Autodesk Inventor part; units mm, degrees
ref_plane "Work Plane3" through (137.521, 56.9702, 137.521) normal (0.7071068, 0, 0.7071068) x (0, -1, 0)
ref_plane "YZ Plane" through (0, 0, 0) normal (1, 0, 0) x (0, 1, 0)
ref_plane "XZ Plane" through (0, 0, 0) normal (0, 1, 0) x (-1, 0, 0)
sketch "Sketch1" plane through (0, 0, 0) normal (0, 0, 1) x (1, 0, 0)
  line L0 (0, 0) -> (0, 228.6)
  line L1 (0, 228.6) -> (76.2, 228.6)
  line L2 (76.2, 228.6) -> (76.2, 219.2528)
  line L3 (76.2, 219.2528) -> (101.6, 219.2528)
  line L4 (101.6, 219.2528) -> (101.6, 0)
  line L5 (101.6, 0) -> (0, 0)
  dimension "d0" = 228.6
  dimension "d1" = 76.2
  dimension "d2" = 9.3472
  dimension "d3" = 25.4
extrude "Extrusion1" add sketch "Sketch1" along normal blind 812.8
sketch "Sketch6" plane through (0, 0, 0) normal (0, -1, 0) x (1, 0, 0)
  line L0 (101.6, 0) -> (101.6, 812.8)
  line L1 (0, 812.8) -> (101.6, 711.2)
  line L2 (76.2038, 736.5962) -> (25.4038, 736.5962)
  line L3 (25.4038, 736.5962) -> (25.4038, 787.3962)
  line L4 (25.4038, 787.3962) -> (76.2, 736.6)
  point P0 (0, 0)
  point P1 (101.6, 101.6)
  dimension "d31" = 35.9156
  dimension "d32" = 50.8
  dimension "d33" = 50.8
extrude "Extrusion4" cut sketch "Sketch6" against normal blind 181.1528
sketch "Sketch7" plane through (25.4038, 0, 736.5962) normal (0, -1, 0) x (1, 0, 0)
  line L0 (76.1962, -634.9962) -> (50.7962, -660.3962)
  line L1 (50.7962, -660.3962) -> (-0.0038, -660.3962)
  line L2 (76.1962, -634.9962) -> (-25.4038, -736.5962)
  line L3 (76.1962, -736.5962) -> (76.1962, 76.2038)
  line L4 (-0.0038, -660.3962) -> (-0.0038, -711.1962)
  line L5 (-0.0038, -711.1962) -> (50.7962, -660.3962)
  point P0 (76.1962, -25.3962)
  dimension "d39" = 50.8
  dimension "d41" = 90
  dimension "d42" = 50.8
extrude "Extrusion5" cut sketch "Sketch7" against normal blind 181.1528
chamfer "Chamfer5" distance 101.6 angle 45 1 edges at (101.6, 109.6264, 812.8)
chamfer "Chamfer6" distance 101.6 angle 45 1 edges at (101.6, 109.6264, 0)
ref_plane "Work Plane3" through (137.521, 56.9702, 137.521) normal (0.7071068, 0, 0.7071068) x (0, -1, 0)
sketch "Sketch9" plane through (137.521, 56.9702, 137.521) normal (0.7071068, 0, 0.7071068) x (0, -1, 0)
  line L0 (-162.2826, 0) -> (-162.2826, -466.9733)
  line L1 (-162.2826, 0) -> (-48.0842, 0)
  line L2 (-162.2826, 0) -> (56.9702, 0)
  dimension "d65" = 114.1984
hole "Hole2" at (137.521, 105.0544, 137.521) direction (-0.7071068, 0, -0.7071068) diameter 12.7 depth 127 tip angle 118
sketch "Sketch10" plane through (0, 181.1528, 0) normal (0, -1, 0) x (1, 0, 0)
  line L0 (76.2, 76.2) -> (76.2, 736.6)
  line L1 (76.2, 76.2) -> (63.5019, 63.5019)
  line L2 (0, 0) -> (76.2, 76.2)
  line L3 (63.5019, 63.5019) -> (38.1019, 63.5019)
  line L4 (38.1019, 63.5019) -> (38.1019, 38.1019)
  line L5 (63.5019, 63.5019) -> (38.1019, 38.1019)
  line L6 (76.2038, 736.5962) -> (63.5058, 749.2942)
  line L7 (63.5058, 749.2942) -> (38.1058, 749.2942)
  line L8 (38.1058, 749.2942) -> (38.1058, 774.6942)
  line L9 (63.5058, 749.2942) -> (38.1058, 774.6942)
  dimension "d73" = 17.9578
  dimension "d74" = 25.4
  dimension "d75" = 17.9578
  dimension "d76" = 25.4
extrude "Extrusion6" cut sketch "Sketch10" against normal blind 3.175 contours L7 L8 L9
sketch "Sketch11" plane through (25.4038, 181.1528, 736.5962) normal (0, -1, 0) x (1, 0, 0)
  line L0 (50.7962, -660.3962) -> (38.0981, -673.0942)
  line L1 (38.0981, -673.0942) -> (12.6962, -673.0942)
  line L2 (12.6962, -673.0942) -> (12.6962, -698.4962)
  line L3 (38.0981, -673.0942) -> (12.6962, -698.4962)
  line L4 (-25.4038, -736.5962) -> (50.7962, -660.3962)
  dimension "d79" = 17.9578
  dimension "d80" = 180
  dimension "d81" = 25.4019
  dimension "d82" = 25.4019
extrude "Extrusion7" cut sketch "Sketch11" against normal blind 3.175
properties part number "SideWidthOutlet" material "Wood (Birch)"
Work out the finished part from the listing and answer in its coordinate system (mm). A direction names the side the tool comes from. Give positions to 0.01 mm unless a question says otherwise; leave off trailing zeros. Loops run counter-clockwise (first coordinate to the right, second up) from the corner with the lowest first, then second, coordinate; pieces in that order, holes last. Notation, with made-up numbers: (73.25, 58) -> (95.25, 58) arc R15 ccw to (95.25, 69) -> close; hole circle Ø4 at (-40, 77.5). An arc over 180 degrees is marked (long way). Use a Markdown table: item, result. Add a question column.
1. Section B-B on x = 8.5 is taken. Determine the outline of the cut face in (y, z).
2. Find the intervals of material crossed by probe 1 along Z at (x, y) = (42.5, 117.5); probe 2 along Y at (x, z) = (92.5, 279.5); probe 3 along Z at (x, y) = (94.5, 90), in increasing order.
3. Flat-ended cylindrical pins translate along their axes: pin 1 Ø4 at (x, y) = (56, 122) entering from +Z; pin 2 Ø1.6 at (x, y) = (49, 182.5) entering from +Z; pin 3 Ø12.5 at (x, z) = (52.5, 45.5) entering from -Y. Find the tip coordinate at first contact, or state that the pin passes through.
4. Determine the mould class of faces 6 (the flat face through (25.4, 89, 51)), 7 (the cylindrical face through (84.17, 104.91, 93.15)), 8 (the flat face through (38, 228.6, 401)), 9 (the flat face through (52, 0, 401)) for opening direction Y: released by +Y, released by -Y, zero draft, split by the parting line, or undercut.
5. Section C-C on y = 210 is taken. Determine the outline of the cut face in (x, z).
6. Section A-A on y = 170.5 is taken. Determine the outline of the cut face in (x, z), and give its area (3 significant figures).
7. For faces 1 (the flat face through (16, 141, 16)), 2 (the flat face through (101.6, 111, 402)), 3 (the flat face through (45, 184.328, 757)), 4 (the flat face through (89, 219.253, 402)), 5 (the flat face through (39, 181.153, 68)), determine the directions among +Z, -Z, +X, -X, +Y, -Y from which every point of the face is accessible in a straight line to the end or side of a thin tool.
Results below:
| question | item | result |
|---|---|---|
| 1 | outline | (0, 8.5) -> (228.6, 8.5) -> (228.6, 804.3) -> (0, 804.3) -> close |
| 2 | probe 1 | z = 76.2 to 736.6 |
| 2 | probe 2 | y = 0 to 219.25 |
| 2 | probe 3 | z = 94.5 to 718.3 |
| 3 | pin 1 | stops at z = 736.6 |
| 3 | pin 2 | stops at z = 749.29 |
| 3 | pin 3 | stops at y = 184.33 |
| 4 | face 6 | zero draft |
| 4 | face 7 | undercut |
| 4 | face 8 | released by +Y |
| 4 | face 9 | released by -Y |
| 5 | outline | (0, 0) -> (101.6, 101.6) -> (101.6, 711.2) -> (0, 812.8) -> close |
| 6 | outline | (0, 0) -> (25.4, 25.4) -> (25.4, 76.2) -> (76.2, 76.2) -> (101.6, 101.6) -> (101.6, 711.2) -> (76.2, 736.6) -> (25.4, 736.6) -> (25.4, 787.4) -> (0, 812.8) -> close |
| 6 | area | 69,700 mm^2 |
| 7 | face 1 | -Z, +X, +Y, -Y |
| 7 | face 2 | +Z, -Z, +X, +Y, -Y |
| 7 | face 3 | +Z, +X, -Y |
| 7 | face 4 | +Z, -Z, +X, +Y |
| 7 | face 5 | -Z, +X, -Y |
